```python
from build123d import *

# Parameters (mm, degrees)
SKETCH1_R           = 2.5
BOSS_EXTRUDE1_DEPTH = 10
SKETCH2_R           = 2.5
BOSS_EXTRUDE2_DEPTH = 10
SKETCH3_R           = 5
SKETCH3_R_2         = 2.5
BOSS_EXTRUDE3_DEPTH = 6
SKETCH4_R           = 2.5
CUT_EXTRUDE1_DEPTH  = 6
CUT_EXTRUDE2_DEPTH  = 41.209967862


with BuildPart() as part:
    # Sketch1 → Boss-Extrude1 (new body)
    with BuildSketch(Plane(origin=(4.043870029, 0, 0), x_dir=(0, 0, -1), z_dir=(1, 0, 0))):
        with BuildLine():
            ThreePointArc((-10.029541992, 0.342879069), (-9.019080639, -0.304016541), (-7.862233613, -0.622153359))
            ThreePointArc((-7.862233613, -0.622153359), (-7.876528296, -1.122077366), (-7.862233613, -1.622001374))
            ThreePointArc((-7.862233613, -1.622001374), (-9.019080639, -1.940138191), (-10.029541992, -2.587033801))
            ThreePointArc((-10.029541992, -2.587033801), (-9.992100042, -2.842856482), (-9.948655897, -3.097728508))
            ThreePointArc((-9.948655897, -3.097728508), (-8.787748306, -3.400713063), (-7.58921172, -3.345793765))
            ThreePointArc((-7.58921172, -3.345793765), (-7.448321757, -3.82566705), (-7.280241692, -4.296705735))
            ThreePointArc((-7.280241692, -4.296705735), (-8.282158911, -4.956757219), (-9.043263028, -5.884241235))
            ThreePointArc((-9.043263028, -5.884241235), (-8.928600062, -6.115972863), (-8.808522437, -6.344945585))
            ThreePointArc((-8.808522437, -6.344945585), (-7.610806331, -6.274360846), (-6.487901298, -5.851761317))
            ThreePointArc((-6.487901298, -5.851761317), (-6.20561798, -6.264610538), (-5.90020538, -6.660655353))
            ThreePointArc((-5.90020538, -6.660655353), (-6.649118154, -7.598011066), (-7.086362862, -8.715294889))
            ThreePointArc((-7.086362862, -8.715294889), (-6.905702889, -8.900251959), (-6.720745819, -9.080911932))
            ThreePointArc((-6.720745819, -9.080911932), (-5.603461996, -8.643667224), (-4.666106283, -7.89475445))
            ThreePointArc((-4.666106283, -7.89475445), (-4.270061468, -8.20016705), (-3.857212247, -8.482450368))
            ThreePointArc((-3.857212247, -8.482450368), (-4.279811776, -9.605355401), (-4.350396515, -10.803071507))
            ThreePointArc((-4.350396515, -10.803071507), (-4.121423793, -10.923149132), (-3.889692165, -11.037812099))
            ThreePointArc((-3.889692165, -11.037812099), (-2.962208149, -10.276707981), (-2.302156665, -9.274790762))
            ThreePointArc((-2.302156665, -9.274790762), (-1.83111798, -9.442870827), (-1.351244695, -9.583760791))
            ThreePointArc((-1.351244695, -9.583760791), (-1.406163992, -10.782297376), (-1.103179437, -11.943204968))
            ThreePointArc((-1.103179437, -11.943204968), (-0.848307411, -11.986649113), (-0.592484731, -12.024091063))
            ThreePointArc((-0.592484731, -12.024091063), (0.054410879, -11.01362971), (0.372547697, -9.856782684))
            ThreePointArc((0.372547697, -9.856782684), (0.872471704, -9.871077366), (1.372395712, -9.856782684))
            ThreePointArc((1.372395712, -9.856782684), (1.690532529, -11.01362971), (2.337428139, -12.024091063))
            ThreePointArc((2.337428139, -12.024091063), (2.59325082, -11.986649113), (2.848122846, -11.943204968))
            ThreePointArc((2.848122846, -11.943204968), (3.151107401, -10.782297376), (3.096188103, -9.583760791))
            ThreePointArc((3.096188103, -9.583760791), (3.576061388, -9.442870827), (4.047100073, -9.274790762))
            ThreePointArc((4.047100073, -9.274790762), (4.707151558, -10.276707981), (5.634635573, -11.037812099))
            ThreePointArc((5.634635573, -11.037812099), (5.866367201, -10.923149132), (6.095339923, -10.803071507))
            ThreePointArc((6.095339923, -10.803071507), (6.024755184, -9.605355401), (5.602155655, -8.482450368))
            ThreePointArc((5.602155655, -8.482450368), (6.015004877, -8.20016705), (6.411049691, -7.89475445))
            ThreePointArc((6.411049691, -7.89475445), (7.348405404, -8.643667224), (8.465689227, -9.080911932))
            ThreePointArc((8.465689227, -9.080911932), (8.650646297, -8.900251959), (8.83130627, -8.715294889))
            ThreePointArc((8.83130627, -8.715294889), (8.394061563, -7.598011066), (7.645148788, -6.660655353))
            ThreePointArc((7.645148788, -6.660655353), (7.950561388, -6.264610538), (8.232844706, -5.851761317))
            ThreePointArc((8.232844706, -5.851761317), (9.355749739, -6.274360846), (10.553465846, -6.344945585))
            ThreePointArc((10.553465846, -6.344945585), (10.67354347, -6.115972863), (10.788206437, -5.884241235))
            ThreePointArc((10.788206437, -5.884241235), (10.02710232, -4.956757219), (9.0251851, -4.296705735))
            ThreePointArc((9.0251851, -4.296705735), (9.193265165, -3.82566705), (9.334155129, -3.345793765))
            ThreePointArc((9.334155129, -3.345793765), (10.532691714, -3.400713063), (11.693599306, -3.097728508))
            ThreePointArc((11.693599306, -3.097728508), (11.737043451, -2.842856482), (11.774485401, -2.587033801))
            ThreePointArc((11.774485401, -2.587033801), (10.764024048, -1.940138191), (9.607177022, -1.622001374))
            ThreePointArc((9.607177022, -1.622001374), (9.621471704, -1.122077366), (9.607177022, -0.622153359))
            ThreePointArc((9.607177022, -0.622153359), (10.764024048, -0.304016541), (11.774485401, 0.342879069))
            ThreePointArc((11.774485401, 0.342879069), (11.737043451, 0.598701749), (11.693599306, 0.853573775))
            ThreePointArc((11.693599306, 0.853573775), (10.532691714, 1.156558331), (9.334155129, 1.101639033))
            ThreePointArc((9.334155129, 1.101639033), (9.193265165, 1.581512318), (9.0251851, 2.052551003))
            ThreePointArc((9.0251851, 2.052551003), (10.02710232, 2.712602487), (10.788206437, 3.640086503))
            ThreePointArc((10.788206437, 3.640086503), (10.67354347, 3.871818131), (10.553465846, 4.100790853))
            ThreePointArc((10.553465846, 4.100790853), (9.355749739, 4.030206114), (8.232844706, 3.607606585))
            ThreePointArc((8.232844706, 3.607606585), (7.950561388, 4.020455806), (7.645148788, 4.416500621))
            ThreePointArc((7.645148788, 4.416500621), (8.394061563, 5.353856334), (8.83130627, 6.471140157))
            ThreePointArc((8.83130627, 6.471140157), (8.650646297, 6.656097227), (8.465689227, 6.8367572))
            ThreePointArc((8.465689227, 6.8367572), (7.348405404, 6.399512492), (6.411049691, 5.650599718))
            ThreePointArc((6.411049691, 5.650599718), (6.015004877, 5.956012318), (5.602155655, 6.238295636))
            ThreePointArc((5.602155655, 6.238295636), (6.024755184, 7.361200669), (6.095339923, 8.558916775))
            ThreePointArc((6.095339923, 8.558916775), (5.866367201, 8.6789944), (5.634635573, 8.793657366))
            ThreePointArc((5.634635573, 8.793657366), (4.707151558, 8.032553249), (4.047100073, 7.03063603))
            ThreePointArc((4.047100073, 7.03063603), (3.576061388, 7.198716095), (3.096188103, 7.339606058))
            ThreePointArc((3.096188103, 7.339606058), (3.151107401, 8.538142644), (2.848122846, 9.699050235))
            ThreePointArc((2.848122846, 9.699050235), (2.59325082, 9.74249438), (2.337428139, 9.779936331))
            ThreePointArc((2.337428139, 9.779936331), (1.690532529, 8.769474978), (1.372395712, 7.612627952))
            ThreePointArc((1.372395712, 7.612627952), (0.872471704, 7.626922634), (0.372547697, 7.612627952))
            ThreePointArc((0.372547697, 7.612627952), (0.054410879, 8.769474978), (-0.592484731, 9.779936331))
            ThreePointArc((-0.592484731, 9.779936331), (-0.848307411, 9.74249438), (-1.103179437, 9.699050235))
            ThreePointArc((-1.103179437, 9.699050235), (-1.406163992, 8.538142644), (-1.351244695, 7.339606058))
            ThreePointArc((-1.351244695, 7.339606058), (-1.83111798, 7.198716095), (-2.302156665, 7.03063603))
            ThreePointArc((-2.302156665, 7.03063603), (-2.962208149, 8.032553249), (-3.889692165, 8.793657366))
            ThreePointArc((-3.889692165, 8.793657366), (-4.121423793, 8.6789944), (-4.350396515, 8.558916775))
            ThreePointArc((-4.350396515, 8.558916775), (-4.279811776, 7.361200669), (-3.857212247, 6.238295636))
            ThreePointArc((-3.857212247, 6.238295636), (-4.270061468, 5.956012318), (-4.666106283, 5.650599718))
            ThreePointArc((-4.666106283, 5.650599718), (-5.603461996, 6.399512492), (-6.720745819, 6.8367572))
            ThreePointArc((-6.720745819, 6.8367572), (-6.905702889, 6.656097227), (-7.086362862, 6.471140157))
            ThreePointArc((-7.086362862, 6.471140157), (-6.649118154, 5.353856334), (-5.90020538, 4.416500621))
            ThreePointArc((-5.90020538, 4.416500621), (-6.20561798, 4.020455806), (-6.487901298, 3.607606585))
            ThreePointArc((-6.487901298, 3.607606585), (-7.610806331, 4.030206114), (-8.808522437, 4.100790853))
            ThreePointArc((-8.808522437, 4.100790853), (-8.928600062, 3.871818131), (-9.043263028, 3.640086503))
            ThreePointArc((-9.043263028, 3.640086503), (-8.282158911, 2.712602487), (-7.280241692, 2.052551003))
            ThreePointArc((-7.280241692, 2.052551003), (-7.448321757, 1.581512318), (-7.58921172, 1.101639033))
            ThreePointArc((-7.58921172, 1.101639033), (-8.787748306, 1.156558331), (-9.948655897, 0.853573775))
            ThreePointArc((-9.948655897, 0.853573775), (-9.992100042, 0.598701749), (-10.029541992, 0.342879069))
        make_face()
        with Locations(Location((0.872471704, -1.122077366, 0), (0, 0, 180))):
            Circle(SKETCH1_R, mode=Mode.SUBTRACT)
    extrude(amount=-BOSS_EXTRUDE1_DEPTH)

    # Sketch2 → Boss-Extrude2 (add)
    with BuildSketch(Plane(origin=(4.043870029, 0, 0), x_dir=(0, 0, -1), z_dir=(1, 0, 0))):
        with BuildLine():
            Line((-2.754400151, 2.319695512), (17.89623712, 24.080926643))
            ThreePointArc((17.89623712, 24.080926643), (24.964881853, 24.266025619), (25.14998083, 17.197380886))
            Line((25.14998083, 17.197380886), (4.499343559, -4.563850245))
            ThreePointArc((4.499343559, -4.563850245), (-2.569301174, -4.748949221), (-2.754400151, 2.319695512))
        make_face()
        with Locations((21.523108975, 20.639153764)):
            Circle(SKETCH2_R, mode=Mode.SUBTRACT)
    extrude(amount=-BOSS_EXTRUDE2_DEPTH)

    # Sketch3 → Boss-Extrude3 (add)
    with BuildSketch(Plane.ZY.offset(5.956129971)):
        with Locations(Location((-21.523108975, 20.639153764, 0), (0, 0, 223.5))):
            Circle(SKETCH3_R)
        with Locations(Location((-21.523108975, 20.639153764, 0), (0, 0, 180))):
            Circle(SKETCH3_R_2, mode=Mode.SUBTRACT)
    extrude(amount=BOSS_EXTRUDE3_DEPTH)

    # Sketch4 → Cut-Extrude1 (cut)
    with BuildSketch(Plane(origin=(4.043870029, 0, 0), x_dir=(0, 0, -1), z_dir=(1, 0, 0))):
        with Locations((0.872471704, -1.122077366)):
            Circle(SKETCH4_R)
    extrude(amount=-CUT_EXTRUDE1_DEPTH, mode=Mode.SUBTRACT)

    # Sketch6 → Cut-Extrude2 (cut, through all)
    with BuildSketch(Plane(origin=(4.043870029, 0, 0), x_dir=(0, 0, -1), z_dir=(1, 0, 0))):
        with BuildLine():
            Line((4.579688985, 10.048212881), (2.187631015, 7.527509733))
            ThreePointArc((2.187631015, 7.527509733), (-2.46576826, 6.965020688), (-6.16100093, 4.08131227))
            Line((-6.16100093, 4.08131227), (-8.58915512, 5.877669916))
            ThreePointArc((-8.58915512, 5.877669916), (-2.68093011, 10.098091069), (4.579688985, 10.048212881))
        make_face()
        with BuildLine():
            Line((11.833432695, 3.164667124), (9.441374725, 0.643963976))
            ThreePointArc((9.441374725, 0.643963976), (9.424184018, -2.969566881), (7.948146758, -6.267932352))
            Line((7.948146758, -6.267932352), (10.39087042, -8.044427405))
            ThreePointArc((10.39087042, -8.044427405), (12.54560297, -2.624359175), (11.833432695, 3.164667124))
        make_face()
    extrude(amount=-CUT_EXTRUDE2_DEPTH, mode=Mode.SUBTRACT)


solid = part.part
```
Check sheet for the modelled part. Datum: model origin and axes. Units: mm. A direction names the side the tool comes from. Round coordinates to 2 decimals unless told otherwise and drop trailing zeros. Order: outer loops, then holes, each group sorted by start corner. A loop starts at its lowest first (then second) coordinate and runs counter-clockwise, first axis right, second up. Notation, with made-up numbers: (73.5, 54.25) -> (83.5, 54.25) arc R13 ccw to (83.5, 63.25) -> close; hole circle Ø1 at (36.5, 30). An arc over 180 degrees is marked (long way). One line per item, written item: value. Start each with the question number.
Q1. Thickness scan on line 1 (Y direction, x = -2.75, z = 8); line 2 (X direction, y = 1, z = 4.5); line 3 (Z direction, x = -5.5, y = 19). Record the ranges inside material, lowest first.
Q2. Set-up check for faces 1 (the face through (-0.9, -3.4, 8.8)), 2 (the face through (-0.89, -7.61, -8.4)), 3 (the face through (-0.89, -7.58, 6.64)), 4 (the face through (-0.886, -10.998, -1.684)), 5 (the face through (4.044, 6, -8)): record each of +Z, -Z, +X, -X, +Y, -Y from which the full face is reachable in a straight line by a thin tool's end or side.
Q3. Cross-section at A-A (y = 21.5). Record the boundary of the cut face in (x, z).
Q4. Mould release check, pull along Z, two halves, no side actions. Record for faces 6 (the face through (-0.886, -1.115, 7.877)), 7 (the face through (-1.956, -1, -1)), 8 (the face through (-0.886, -9.589, 4.276)), 9 (the face through (-11.956, 18, -21)): pulls with the +Z half, pulls with the -Z half, needs draft (parallel to the pull), parting line crosses it, or undercut.
Q5. Gauge pin test, flat ends, axial feed: pin 1 Ø6 at (y, z) = (12.5, -7) entering from -X; pin 2 Ø6 at (y, z) = (20.64, -21.52) entering from +X; pin 3 Ø6 at (x, y) = (2, -4) entering from -Z; pin 4 Ø3 at (x, z) = (2.5, -12) entering from -Y. Record the tip position at first contact, or that the pin passes through.
Q6. Cross-section at B-B (z = -17). Record the boundary of the cut face in (x, y), and give its area (3 significant figures).
Q7. Cross-section at D-D (x = -1). Give the number of separate pieces and of enclosed holes in the cut face, and give its area (3 significant figures).
Q8. Cross-section at C-C (x = -7.75). Record the boundary of the cut face in (y, z).
Completed:
1. line 1: y = -6.34 to -4.73, -3.41 to -1.64, -0.6 to 1.16, 2.48 to 4.09
1. line 2: x = -5.96 to 4.04
1. line 3: z = -26.25 to -23.41, -19.64 to -13.07
2. face 1: +X, -X
2. face 2: -Z, +X, -X
2. face 3: +Z, +X, -X
2. face 4: +X, -X, -Y
2. face 5: +Z, -Z, +X, +Y, -Y
3. outline: (-11.96, -26.45) -> (4.04, -26.45) -> (4.04, -23.87) -> (-11.96, -23.87) -> close; (-11.96, -19.18) -> (4.04, -19.18) -> (4.04, -15.45) -> (-5.96, -15.45) -> (-5.96, -16.6) -> (-11.96, -16.6) -> close
4. face 6: pulls with the +Z half
4. face 7: undercut
4. face 8: undercut
4. face 9: needs draft
5. pin 1: stops at x = -5.96
5. pin 2: stops at x = 4.04
5. pin 3: stops at z = -9.62
5. pin 4: stops at y = 1.76
6. outline: (-11.96, 18.51) -> (-5.96, 18.51) -> (-5.96, 8.61) -> (4.04, 8.61) -> (4.04, 23.14) -> (-5.96, 23.14) -> (-5.96, 22.77) -> (-11.96, 22.77) -> close
6. area: 171 mm²
7. separate pieces: 1
7. enclosed holes: 2
7. area: 489 mm²
8. outline: circle Ø10 at (20.64, -21.52); hole circle Ø5 at (20.64, -21.52)
